Autodesk Inventor part; units mm, degrees
ref_plane "YZ Plane" through (0, 0, 0) normal (1, 0, 0) x (0, 1, 0)
ref_plane "XZ Plane" through (0, 0, 0) normal (0, 1, 0) x (-1, 0, 0)
ref_plane "XY Plane" through (0, 0, 0) normal (0, 0, 1) x (1, 0, 0)
sketch "スケッチ1" plane through (0, 0, 0) normal (0, 1, 0) x (-1, 0, 0)
  line L0 (0, 0) -> (260, 0)
  line L1 (260, 0) -> (260, 60)
  line L2 (260, 60) -> (0, 60)
  line L3 (0, 60) -> (0, 0)
  dimension "d0" = 260
  dimension "d1" = 60
extrude "押し出し1" add sketch "スケッチ1" along normal blind 2
sketch "スケッチ2" plane through (0, 0, 0) normal (0, 1, 0) x (-1, 0, 0)
  circle A0 centre (30, 30) radius 12
  line L0 (0, 60) -> (0, 0)
  line L1 (0, 0) -> (260, 0)
  dimension "d4" = 24
  dimension "d5" = 30
  dimension "d6" = 30
extrude "押し出し2" cut sketch "スケッチ2" along normal blind 10
sketch "スケッチ3" plane through (0, 2, 0) normal (0, 1, 0) x (1, 0, 0)
  circle A0 centre (-30, -30) radius 12
  circle A1 centre (-30, -13) radius 2
  circle A2 centre (-13, -30) radius 2
  circle A3 centre (-47, -30) radius 2
  circle A4 centre (-30, -47) radius 2
  point P0 (0, 0)
  dimension "d10" = 4
  dimension "d11" = 4
  dimension "d12" = 4
  dimension "d13" = 4
extrude "押し出し3" cut sketch "スケッチ3" against normal blind 10 contours A1 | A2 | A3 | A4
sketch "スケッチ4" plane through (0, 0, 0) normal (0, -1, 0) x (1, 0, 0)
  circle A0 centre (-230, 30) radius 11.5
  line L0 (-260, 0) -> (-260, 60)
  point P0 (0, 0)
  dimension "d16" = 23
  dimension "d26" = 30
extrude "押し出し4" cut sketch "スケッチ4" against normal blind 10
sketch "スケッチ5" plane through (0, 0, 0) normal (0, -1, 0) x (1, 0, 0)
  circle A0 centre (-230, 30) radius 11.5
  circle A1 centre (-246, 30) radius 2.25
  circle A2 centre (-230, 46) radius 2.25
  circle A3 centre (-214, 30) radius 2.25
  circle A4 centre (-230, 14) radius 2.25
  point P0 (0, 0)
  dimension "d28" = 4.5
  dimension "d29" = 4.5
  dimension "d30" = 4.5
  dimension "d31" = 4.5
extrude "押し出し6" cut sketch "スケッチ5" against normal blind 10 contours A1 | A2 | A3 | A4
sketch "スケッチ6" plane through (0, 0, 0) normal (0, -1, 0) x (1, 0, 0)
  circle A0 centre (-158, 10) radius 2.6
  line L0 (0, 0) -> (-260, 0)
  circle A1 centre (-150, 10) radius 2.6
  circle A2 centre (-110, 10) radius 2.6
  circle A3 centre (-102, 10) radius 2.6
  circle A4 centre (-158, 50) radius 2.6
  line L1 (-260, 60) -> (0, 60)
  circle A5 centre (-150, 50) radius 2.6
  circle A6 centre (-110, 50) radius 2.6
  circle A7 centre (-102, 50) radius 2.6
  line L2 (-260, 0) -> (-260, 60)
  dimension "d34" = 5.2
  dimension "d35" = 10
  dimension "d36" = 5.2
  dimension "d37" = 8
  dimension "d38" = 5.2
  dimension "d39" = 40
  dimension "d40" = 5.2
  dimension "d41" = 8
  dimension "d42" = 5.2
  dimension "d43" = 10
  dimension "d44" = 5.2
  dimension "d45" = 5.2
  dimension "d46" = 5.2
  dimension "d49" = 102
  dimension "d50" = 40
  dimension "d51" = 8
  dimension "d52" = 8
  dimension "d53" = 102
extrude "押し出し7" cut sketch "スケッチ6" against normal blind 10
properties part number "UpperArm1" material "アルミニウム 6061"
Could you check a few things on this model? Use its own coordinates, in mm. Give positions to 0.01 mm unless a question says otherwise; leave off trailing zeros. Order: outer loops, then holes, each group sorted by start corner. A loop starts at its lowest first (then second) coordinate and runs counter-clockwise, first axis right, second up. Notation, with made-up numbers: (3.25, 55.25) - (16.25, 55.25) arc R28 cw to (16.25, 73.25) - close; hole circle Ø1 at (62, 58.5). An arc over 180 degrees is marked (long way). One line per question, with ' | ' between items. Start each with the question number.
Item 1: I want a section at B-B on z = 36.5. Write out the boundary of the cut face in (x, y), then the cut area to 3 significant figures.
Item 2: I need wall thicknesses on probe 1 along Z at (x, y) = (-150, 1.05); probe 2 along Z at (x, y) = (-230, 0.9); probe 3 along Z at (x, y) = (-30, 0.9). Which ranges of each line are inside material? Lowest first, please. Write a range as [from, to].
Item 3: I want a section at A-A on x = -158. Write out the boundary of the cut face in (y, z), then the cut area to 3 significant figures.
Item 4: I want a section at C-C on x = -223.5. Write out the boundary of the cut face in (y, z), then the cut area to 3 significant figures.
Item 5: Thinking about a two-plate mould opening in Z: for faces 1 (the flat face through (-128, 2, 30)), 2 (the cylindrical face through (-248.248, 0.986, 30.099)), which applies, pulls with the +Z half, pulls with the -Z half, needs draft (parallel to the pull), parting line crosses it, or undercut?
Verdict:
1) outline: (-260, 0) - (-239.49, 0) - (-239.49, 2) - (-260, 2) - close; (-220.51, 0) - (-40.09, 0) - (-40.09, 2) - (-220.51, 2) - close; (-19.91, 0) - (0, 0) - (0, 2) - (-19.91, 2) - close | area: 442 mm^2
2) probe 1: [0, 7.4], [12.6, 47.4], [52.6, 60] | probe 2: [0, 11.75], [16.25, 18.5], [41.5, 43.75], [48.25, 60] | probe 3: [0, 11], [15, 18], [42, 45], [49, 60]
3) outline: (0, 0) - (2, 0) - (2, 7.4) - (0, 7.4) - close; (0, 12.6) - (2, 12.6) - (2, 47.4) - (0, 47.4) - close; (0, 52.6) - (2, 52.6) - (2, 60) - (0, 60) - close | area: 99.2 mm^2
4) outline: (0, 0) - (2, 0) - (2, 20.51) - (0, 20.51) - close; (0, 39.49) - (2, 39.49) - (2, 60) - (0, 60) - close | area: 82.1 mm^2
5) face 1: needs draft | face 2: undercut
